For this review, use the dimensioned drawing (mm, ordinates from the lowest corner) and the shaded views. Round coordinates to 2 decimals unless told otherwise and drop trailing zeros. Loops run counter-clockwise (first coordinate to the right, second up) from the corner with the lowest first, then second, coordinate; pieces in that order, holes last. Notation, with made-up numbers: (-33.5, 46.25) - (10.5, 46.25) arc R16 ccw to (10.5, 55.25) - close; hole circle Ø11 at (22, -17). An arc over 180 degrees is marked (long way). Return JSON: item names as keys, results as strings. Group by question number.
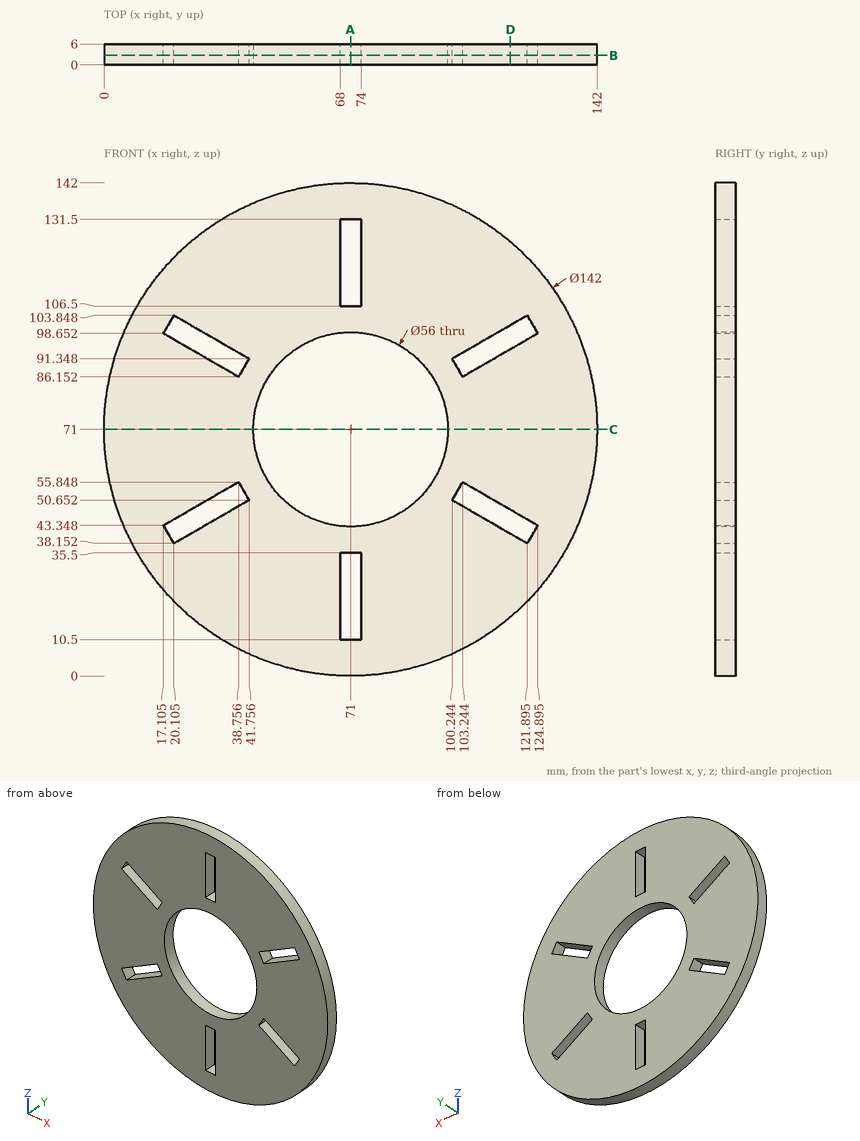
Q1. Add section A-A, the plane x = 71. State the section outline as (y, z) points.
Q2. Insertion check: pin 1 Ø3 at (x, y) = (59.5, 1) entering from +Z; pin 2 Ø3 at (x, y) = (106, 1) entering from +Z; pin 3 Ø3 at (x, y) = (72, 4.5) entering from +Z. Each pin has a flat end and moves straight along its axis. Give the tip position at first contact, or say it passes through.
Q3. Add section C-C, the plane z = 71. State the section outline as (x, y) points, plus the area to 3 significant figures.
Q4. Add section B-B, the plane y = 2.75. State the section outline as (x, z) points (1 decimal), plus the area to 3 significant figures.
Q5. For line 1 (Z direction, x = 70.5, y = 3.25) (1 decimal); line 2 (X direction, y = 4.35, z = 71); line 3 (Z direction, x = 30.5, y = 3) (1 decimal), list the stretches that pass through material, from the lowest coordinate up.
Q6. Add section D-D, the plane x = 117. State the section outline as (y, z) points, plus the area to 3 significant figures.
Evaluation:
{
 "1": {"outline": "(0, 0) - (6, 0) - (6, 10.5) - (0, 10.5) - close; (0, 35.5) - (6, 35.5) - (6, 43) - (0, 43) - close; (0, 99) - (6, 99) - (6, 106.5) - (0, 106.5) - close; (0, 131.5) - (6, 131.5) - (6, 142) - (0, 142) - close"},
 "2": {"pin 1": "z = 141.29", "pin 2": "z = 133.6", "pin 3": "z = 142"},
 "3": {"outline": "(0, 0) - (43, 0) - (43, 6) - (0, 6) - close; (99, 0) - (142, 0) - (142, 6) - (99, 6) - close", "area": "516 mm²"},
 "4": {"outline": "circle Ø142 at (71, 71); hole (17.1, 43.3) - (20.1, 38.2) - (41.8, 50.7) - (38.8, 55.8) - close; hole (17.1, 98.7) - (38.8, 86.2) - (41.8, 91.3) - (20.1, 103.8) - close; hole circle Ø56 at (71, 71); hole (68, 10.5) - (74, 10.5) - (74, 35.5) - (68, 35.5) - close; hole (68, 106.5) - (74, 106.5) - (74, 131.5) - (68, 131.5) - close; hole (100.2, 50.7) - (121.9, 38.2) - (124.9, 43.3) - (103.2, 55.8) - close; hole (100.2, 91.3) - (103.2, 86.2) - (124.9, 98.7) - (121.9, 103.8) - close", "area": "12,500 mm²"},
 "5": {"line 1": "0 to 10.5, 35.5 to 43, 99 to 106.5, 131.5 to 142", "line 2": "0 to 43, 99 to 142", "line 3": "12.7 to 44.2, 51.1 to 90.9, 97.8 to 129.3"},
 "6": {"outline": "(0, 16.92) - (6, 16.92) - (6, 40.98) - (0, 40.98) - close; (0, 47.91) - (6, 47.91) - (6, 94.09) - (0, 94.09) - close; (0, 101.02) - (6, 101.02) - (6, 125.08) - (0, 125.08) - close", "area": "566 mm²"}
}
